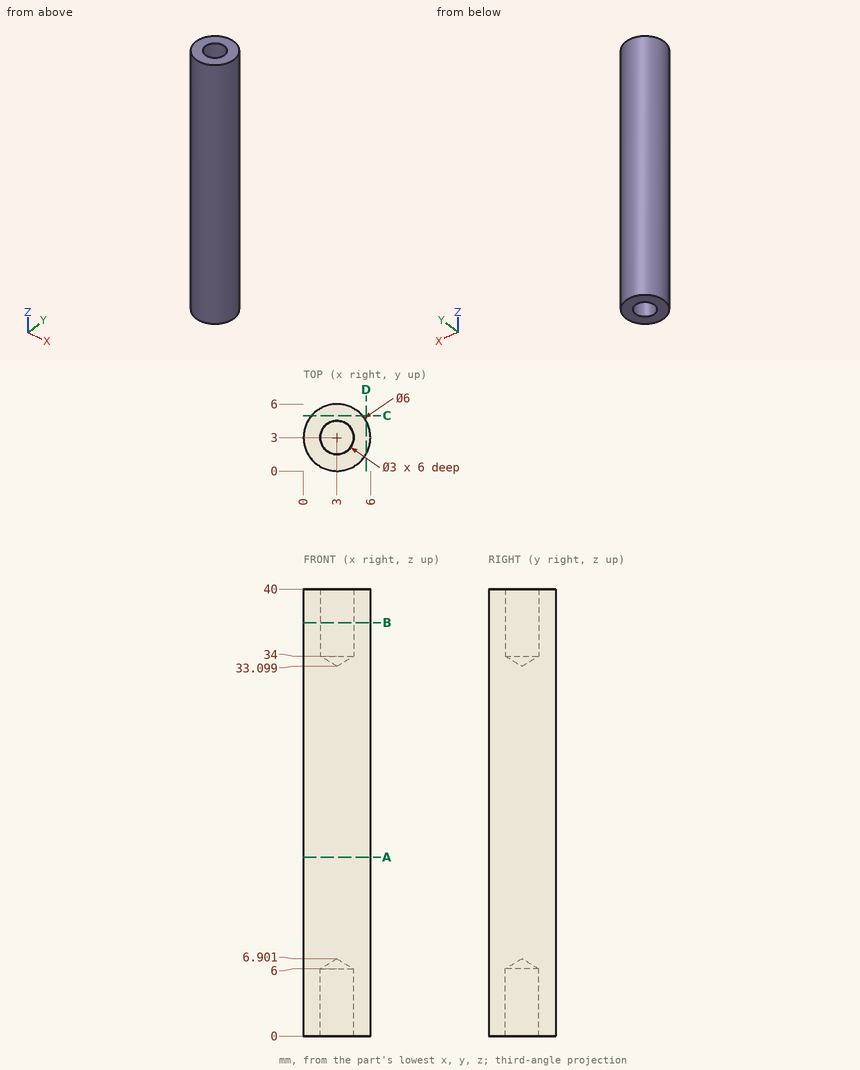
Geometry check sheet. Reference: drawing and pictorial views, mm from the part's lowest x, y, z. Give positions to 0.01 mm unless a question says otherwise; leave off trailing zeros. Loops run counter-clockwise (first coordinate to the right, second up) from the corner with the lowest first, then second, coordinate; pieces in that order, holes last. Notation, with made-up numbers: (25, 2) - (36, 2) arc R24 ccw to (36, 26) - close; hole circle Ø11 at (11.5, 77.25). An arc over 180 degrees is marked (long way). One line per question, with ' | ' between items. Start each with the question number.
1. Material ranges on line 1 along Y through (x, z) = (3, 36.65); line 2 along X through (y, z) = (0.4, 19) (1 decimal); line 3 along X through (y, z) = (4.8, 16), recorded low to high. Write a range as [from, to].
2. Cross-section at D-D, the plane x = 5.6. Enter the section's corners in (y, z).
3. Cross-section at A-A, the plane z = 16. Enter the section's corners in (x, y), plus the area to 3 significant figures.
4. Cross-section at B-B, the plane z = 37. Enter the section's corners in (x, y).
5. Gauge pin test, flat ends, axial feed: pin 1 Ø3 at (x, y) = (1.5, 1.5) entering from -Z; pin 2 Ø1 at (x, y) = (3.5, 3) entering from -Z; pin 3 Ø2.5 at (x, y) = (3, 3) entering from +Z; pin 4 Ø1 at (y, z) = (4, 22.5) entering from -X. Record the tip position at first contact, or that the pin passes through.
6. Cross-section at C-C, the plane y = 4.95. Enter the section's corners in (x, z).
Check result:
1) line 1: y = [0, 1.5], [4.5, 6] | line 2: x = [1.5, 4.5] | line 3: x = [0.6, 5.4]
2) outline: (1.5, 0) - (4.5, 0) - (4.5, 40) - (1.5, 40) - close
3) outline: circle Ø6 at (3, 3) | area: 28.3 mm2
4) outline: circle Ø6 at (3, 3); hole circle Ø3 at (3, 3)
5) pin 1: stops at z = 0 | pin 2: stops at z = 6.3 | pin 3: stops at z = 33.85 | pin 4: stops at x = 0.04
6) outline: (0.72, 0) - (5.28, 0) - (5.28, 40) - (0.72, 40) - close
